For this review, take the finished solid that the model builds, in its own axes (mm). A direction names the side the tool comes from. Give positions to 0.01 mm unless a question says otherwise; leave off trailing zeros. Write item = value, one per line.
```python
from build123d import *

# Parameters (mm, degrees)
SKETCH2_R           = 1.892615742
SKETCH2_R_2         = 1.931502603
SKETCH2_R_3         = 1.328987324
SKETCH2_R_4         = 1.256139718
SKETCH2_R_5         = 2.25
SKETCH2_R_6         = 1.346221639
SKETCH2_R_7         = 1.388588177
SKETCH2_W           = 5.927
SKETCH2_H           = 5.645543841
SKETCH2_H_2         = 5.614229543
SKETCH2_H_3         = 5.725940204
SKETCH2_H_4         = 5.592813932
BOSS_EXTRUDE3_DEPTH = 5


with BuildPart() as part:
    # Sketch2 → Boss-Extrude3 (new body)
    with BuildSketch(Plane.XY):
        with BuildLine():
            Line((185, -142.659400732), (185, -37.931368938))
            ThreePointArc((185, -37.931368938), (182.071067812, -30.860301126), (175, -27.931368938))
            Line((175, -27.931368938), (10, -27.931368938))
            ThreePointArc((10, -27.931368938), (2.928932188, -30.860301126), (0, -37.931368938))
            Line((0, -37.931368938), (0, -142.659400732))
            ThreePointArc((0, -142.659400732), (2.928932188, -149.730468544), (10, -152.659400732))
            Line((10, -152.659400732), (175, -152.659400732))
            ThreePointArc((175, -152.659400732), (182.071067812, -149.730468544), (185, -142.659400732))
        make_face()
        with Locations((154.694647781, -42.076845181)):
            Circle(SKETCH2_R, mode=Mode.SUBTRACT)
        with Locations((154.690357003, -70.942028449)):
            Circle(SKETCH2_R_2, mode=Mode.SUBTRACT)
        with Locations((113.33050486, -94.586932903)):
            Circle(SKETCH2_R_3, mode=Mode.SUBTRACT)
        with Locations((168.03050486, -88.730534378)):
            Circle(SKETCH2_R_4, mode=Mode.SUBTRACT)
        with Locations((22.757067444, -122.885983842)):
            Circle(SKETCH2_R_5, mode=Mode.SUBTRACT)
        with Locations((113.33050486, -120.963520008)):
            Circle(SKETCH2_R_6, mode=Mode.SUBTRACT)
        with Locations((168.03050486, -138.230534378)):
            Circle(SKETCH2_R_7, mode=Mode.SUBTRACT)
        with Locations((87.938265458, -122.885983842)):
            Circle(SKETCH2_R_5, mode=Mode.SUBTRACT)
        with Locations((87.938265458, -57.704785828)):
            Circle(SKETCH2_R_5, mode=Mode.SUBTRACT)
        with Locations((22.757067444, -57.704785828)):
            Circle(SKETCH2_R_5, mode=Mode.SUBTRACT)
        with Locations((166.691794259, -42.169597018)):
            Rectangle(SKETCH2_W, SKETCH2_H, mode=Mode.SUBTRACT)
        with Locations((142.703794259, -42.185254167)):
            Rectangle(SKETCH2_W, SKETCH2_H_2, mode=Mode.SUBTRACT)
        with Locations((166.691794259, -70.915398836)):
            Rectangle(SKETCH2_W, SKETCH2_H_3, mode=Mode.SUBTRACT)
        with Locations((142.703794259, -70.981961972)):
            Rectangle(SKETCH2_W, SKETCH2_H_4, mode=Mode.SUBTRACT)
        Polygon((10.446338383, -114.181499366), (14.68897907, -118.424140053), (18.295223654, -114.817895469), (14.052582967, -110.575254782), align=None, mode=Mode.SUBTRACT)
        Polygon((35.067796504, -131.590468319), (30.825155817, -127.347827632), (27.218911233, -130.954072216), (31.46155192, -135.196712903), align=None, mode=Mode.SUBTRACT)
        Polygon((96.642749934, -110.575254782), (92.400109247, -114.817895469), (96.006353831, -118.424140053), (100.248994518, -114.181499366), align=None, mode=Mode.SUBTRACT)
        Polygon((79.233780981, -135.196712903), (83.476421669, -130.954072216), (79.870177084, -127.347827632), (75.627536397, -131.590468319), align=None, mode=Mode.SUBTRACT)
        Polygon((75.627536397, -49.000301352), (79.870177084, -53.242942039), (83.476421669, -49.636697455), (79.233780981, -45.394056768), align=None, mode=Mode.SUBTRACT)
        Polygon((100.248994518, -66.409270305), (96.006353831, -62.166629618), (92.400109247, -65.772874202), (96.642749934, -70.015514889), align=None, mode=Mode.SUBTRACT)
        Polygon((31.46155192, -45.394056768), (27.218911233, -49.636697455), (30.825155817, -53.242942039), (35.067796504, -49.000301352), align=None, mode=Mode.SUBTRACT)
        Polygon((14.052582967, -70.015514889), (18.295223654, -65.772874202), (14.68897907, -62.166629618), (10.446338383, -66.409270305), align=None, mode=Mode.SUBTRACT)
    extrude(amount=BOSS_EXTRUDE3_DEPTH)


solid = part.part
```
1. Machinability: for faces 3 (the face through (94, -27.931, 2)), 4 (the face through (143, -73.778, 2)), which of the approach directions +Z, -Z, +X, -X, +Y, -Y give a long, thin tool a straight path to every point of the face, cutting with its end or side? Answer none if there is none.
Responses:
face_3 = +Z, -Z, +X, -X, +Y
face_4 = +Z, -Z
2. The part is to be moulded in two halves that separate along Y. For faces 1 (the face through (139.74, -71, 2)), 2 (the face through (182.15, -30.94, 2.46)), say which applies: +Y half, -Y half, draft (parallel to the pull), parting line (faces both ways), or undercut.
Responses:
face_1 = undercut
face_2 = +Y half
3. We need section A-A, the plane z = 0.85. Count the separate pieces of the cut face and the enclosed holes in it, then the cut area to 3 significant figures.
Responses:
separate_pieces = 1
enclosed_holes = 22
area = 22,500 mm2
4. Insertion check: P1, Ø4.5, axis at x = 113.33, y = -94.59, coming from the +Z side. The pin has a flat end and moves straight along its axis. Give the tip position at first contact, or say it passes through.
Responses:
P1 = 5
5. For line 1 along Y through (x, z) = (143.5, 3.7); line 2 along X through (y, z) = (-111, 4.5); line 3 along Y through (x, z) = (12.5, 2.4), list the stretches that pass through material, from the lowest coordinate up. Write a range as from..to.
Responses:
line_1 = -152.66..-73.78, -68.19..-44.99, -39.38..-27.93
line_2 = 0..13.63, 14.48..96.22, 97.07..185
line_3 = -152.66..-116.24, -112.13..-68.46, -64.36..-27.93
